Could you check a few things on this drawing? It's one solid part, dimensions in mm from its lowest x, y, z. A direction names the side the tool comes from. Give positions to 0.01 mm unless a question says otherwise; leave off trailing zeros. Order: outer loops, then holes, each group sorted by start corner. A loop starts at its lowest first (then second) coordinate and runs counter-clockwise, first axis right, second up.
(1) Imagine slicing it at B-B, the plane y = 26.2. Write out the boundary of the cut face in (x, z), then the cut area to 3 significant figures.
(2) Imagine slicing it at D-D, the plane y = 36.5. Write out the boundary of the cut face in (x, z) (1 decimal).
(3) Imagine slicing it at A-A, the plane x = 7.25. Write out the boundary of the cut face in (y, z), then the cut area to 3 significant figures.
(4) If I drill on probe 1 along X at (y, z) = (25, 7.5); probe 2 along Z at (x, y) = (7.5, 9); probe 3 along Z at (x, y) = (21, 3), over which ranges is the centre line in solid material (lowest first)?
(5) Will these pins go through, and if not, where does the flat tip stop? pin 1 (12.5 mm diameter, centred on y = 26.2, z = 20, fed in from +X); pin 2 (7.5 mm diameter, centred on x = 12, z = 2.5, fed in from -Y); pin 3 (1 mm diameter, centred on y = 40, z = 19.5, fed in from +X).
(6) If we mould it in two halves opening along Z, with no side actions, what happens to the marked faces 4, 5, 6 and 7? For each: released by +Z, released by -Z, zero draft, split by the parting line, or undercut.
(7) Imagine slicing it at C-C, the plane z = 28. Write out the boundary of the cut face in (x, y).
(8) On a 3-axis mill with a long thin cutter (end or side, diameter ignored), from which of +Z, -Z, +X, -X, +Y, -Y can I reach the whole of each face in a straight line? I mean the marked faces 1, 2 and 3. Say none if no direction works.
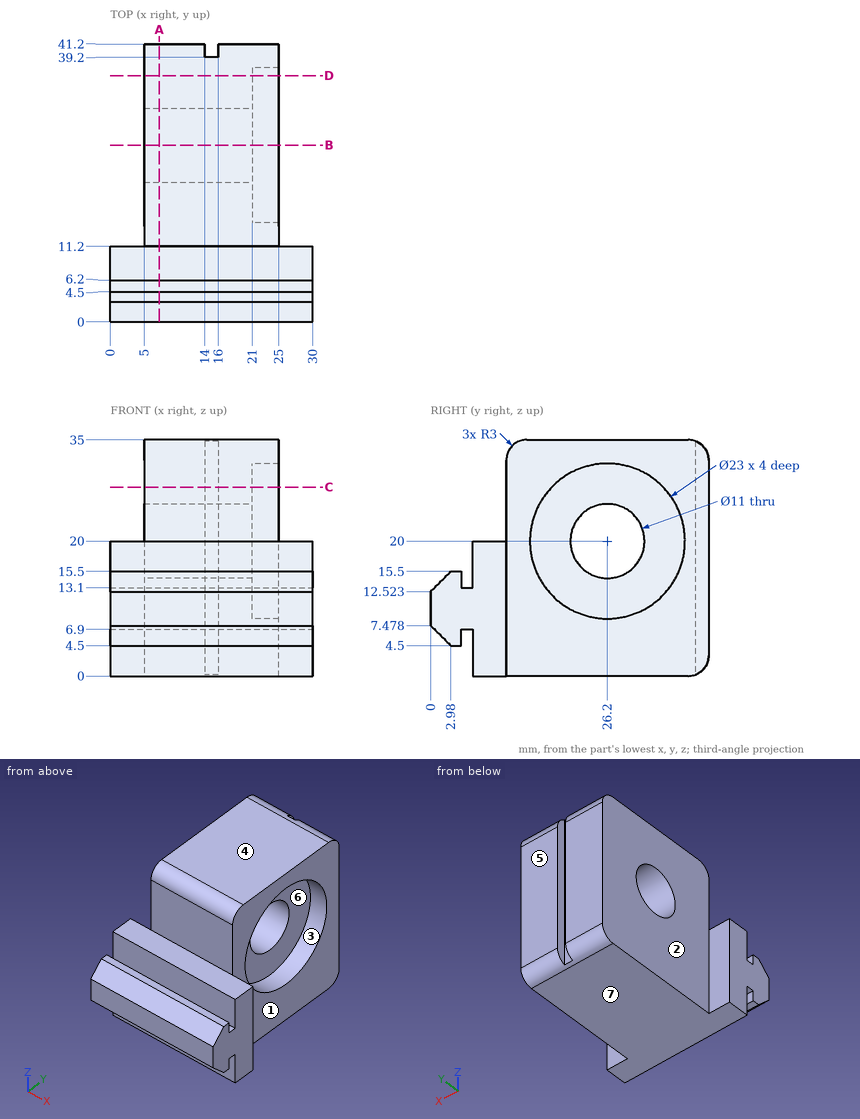
Answer block:
1. outline: (5, 0) - (25, 0) - (25, 8.5) - (21, 8.5) - (21, 14.5) - (5, 14.5) - close; (5, 25.5) - (21, 25.5) - (21, 31.5) - (25, 31.5) - (25, 35) - (5, 35) - close
1. area: 432 mm2
2. outline: (5, 0) - (25, 0) - (25, 14.9) - (21, 14.9) - (21, 25.1) - (25, 25.1) - (25, 35) - (5, 35) - close
3. outline: (0, 7.48) - (2.98, 4.5) - (4.5, 4.5) - (4.5, 6.9) - (6.2, 6.9) - (6.2, 0) - (38.2, 0) arc R3 ccw to (41.2, 3) - (41.2, 32) arc R3 ccw to (38.2, 35) - (14.2, 35) arc R3 ccw to (11.2, 32) - (11.2, 20) - (6.2, 20) - (6.2, 13.1) - (4.5, 13.1) - (4.5, 15.5) - (2.98, 15.5) - (0, 12.52) - close; hole circle Ø11 at (26.2, 20)
3. area: 1,100 mm2
4. probe 1: x = 5 to 25
4. probe 2: z = 0 to 20
4. probe 3: z = 4.5 to 15.5
5. pin 1: stops at x = 21
5. pin 2: stops at y = 1.23
5. pin 3: stops at x = 25
6. face 4: released by +Z
6. face 5: zero draft
6. face 6: undercut
6. face 7: released by -Z
7. outline: (5, 11.2) - (25, 11.2) - (25, 17.94) - (21, 17.94) - (21, 34.46) - (25, 34.46) - (25, 41.2) - (16, 41.2) - (16, 39.2) - (14, 39.2) - (14, 41.2) - (5, 41.2) - close
8. face 1: +Z, -Z, +X, +Y
8. face 2: +Z, -Z, -X, +Y
8. face 3: +X
